Here's the drawing with two shaded views (mm, measured from the low corner). I have some questions. A direction names the side the tool comes from. Give positions to 0.01 mm unless a question says otherwise; leave off trailing zeros. Loops run counter-clockwise (first coordinate to the right, second up) from the corner with the lowest first, then second, coordinate; pieces in that order, holes last.
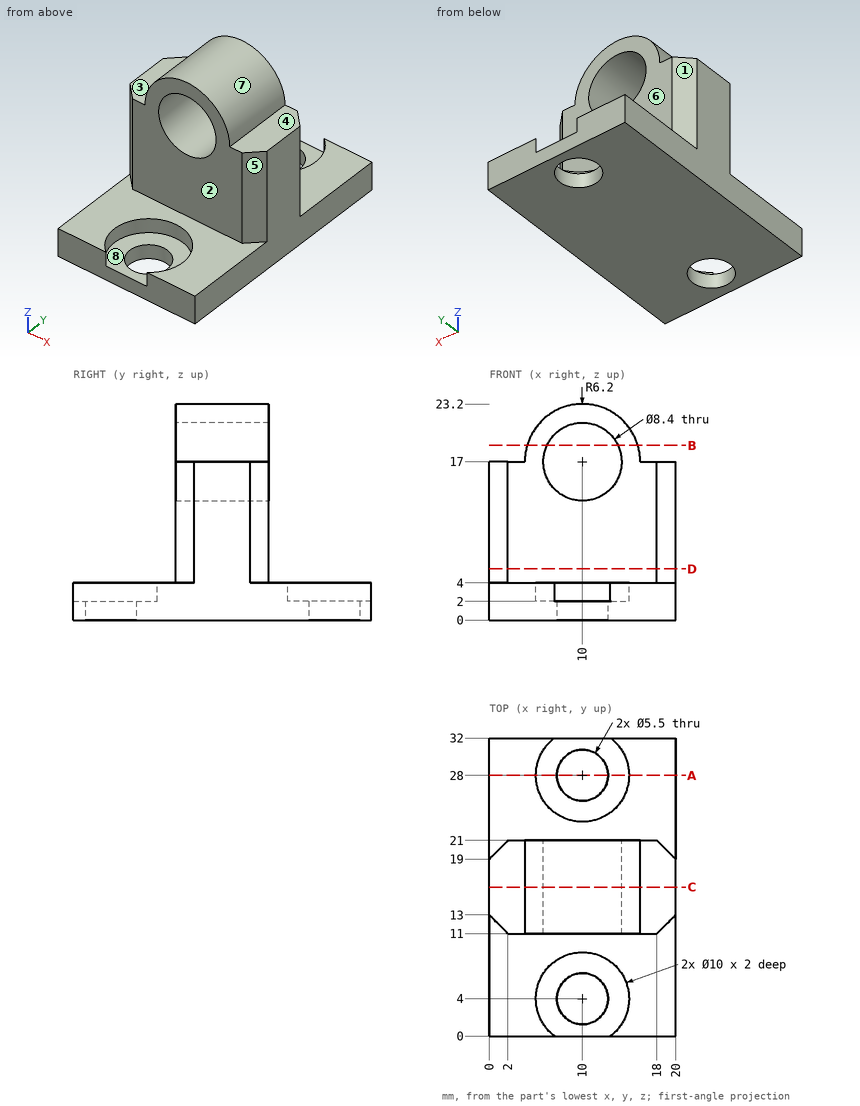
(1) Will these pins go through, and if not, where does the flat tip stop? P1, Ø3, axis at x = 18, y = 14, coming from the +Z side; P2, Ø10.5, axis at x = 13, y = 4, coming from the +Z side; P3, Ø2, axis at x = 11, z = 5.5, coming from the +Y side.
Returned:
P1: stops at z = 17
P2: stops at z = 4
P3: stops at y = 21
(2) Thinking about a two-plate mould opening in Y: for the marked faces 5, 6, 7 and 8, which applies, pulls with the +Y half, pulls with the -Y half, needs draft (parallel to the pull), parting line crosses it, or undercut?
Returned:
face 5: pulls with the -Y half
face 6: pulls with the +Y half
face 7: needs draft
face 8: undercut
(3) Which directions (+Z, -Z, +X, -X, +Y, -Y) give clear straight access to the entire face, cutting with the end or side of a thin tool? Please do the marked faces 1, 2, 3 and 4.
Returned:
face 1: +Z, -X, +Y
face 2: +Z, +X, -X, -Y
face 3: +Z, -X, +Y, -Y
face 4: +Z, +X, +Y, -Y
(4) Suppose I cut it at A-A on y = 28. List the corners of the cut face in (x, z) for me.
Returned:
outline: (0, 0) - (7.25, 0) - (7.25, 2) - (5, 2) - (5, 4) - (0, 4) - close; (12.75, 0) - (20, 0) - (20, 4) - (15, 4) - (15, 2) - (12.75, 2) - close
(5) Suppose I cut it at C-C on y = 16. List the corners of the cut face in (x, z) for me, plus the area to 3 significant figures.
Returned:
outline: (0, 0) - (20, 0) - (20, 17) - (16.2, 17) arc R6.2 ccw to (3.8, 17) - (0, 17) - close; hole circle Ø8.4 at (10, 17)
area: 345 mm2
(6) Please list where these lines run through material, in increasing order: probe 1 along Y at (x, z) = (10, 0.9); probe 2 along X at (y, z) = (4, 0.85); probe 3 along X at (y, z) = (28, 2.55).
Returned:
probe 1: y = 0 to 1.25, 6.75 to 25.25, 30.75 to 32
probe 2: x = 0 to 7.25, 12.75 to 20
probe 3: x = 0 to 5, 15 to 20
(7) Suppose I cut it at B-B on z = 18.75. List the corners of the cut face in (x, y) for me, plus the area to 3 significant figures.
Returned:
outline: (4.05, 11) - (6.18, 11) - (6.18, 21) - (4.05, 21) - close; (13.82, 11) - (15.95, 11) - (15.95, 21) - (13.82, 21) - close
area: 42.6 mm2
(8) Suppose I cut it at D-D on z = 5.5. List the corners of the cut face in (x, y) for me.
Returned:
outline: (0, 13) - (2, 11) - (18, 11) - (20, 13) - (20, 19) - (18, 21) - (2, 21) - (0, 19) - close
